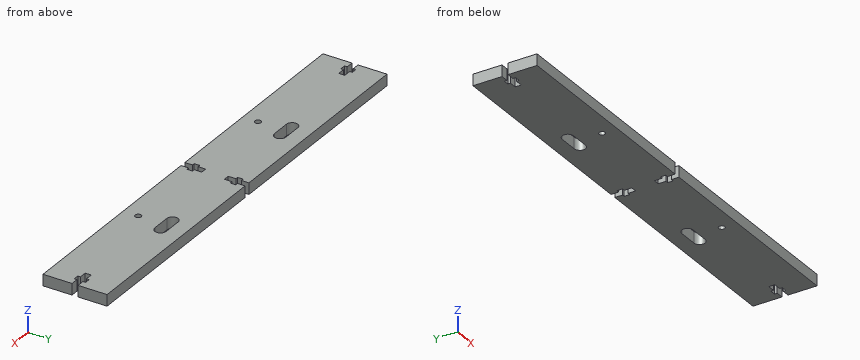
```python
from build123d import *

# Parameters (mm, degrees)
ESBO_O1_R                = 1.6
RESSALTO_EXTRUS_O1_DEPTH = 6


with BuildPart() as part:
    # Esboço1 → Ressalto-extrusão1 (new body)
    with BuildSketch(Plane.XY):
        Polygon((117, 17), (117, 1.6), (113, 1.6), (113, 3), (110, 3), (110, 1.6), (106, 1.6), (106, -1.6), (110, -1.6), (110, -3), (113, -3), (113, -1.6), (117, -1.6), (117, -17), (1.6, -17), (1.6, -13), (3, -13), (3, -10), (1.6, -10), (1.6, -6), (-1.6, -6), (-1.6, -10), (-3, -10), (-3, -13), (-1.6, -13), (-1.6, -17), (-117, -17), (-117, -1.6), (-113, -1.6), (-113, -3), (-110, -3), (-110, -1.6), (-106, -1.6), (-106, 1.6), (-110, 1.6), (-110, 3), (-113, 3), (-113, 1.6), (-117, 1.6), (-117, 17), (-1.6, 17), (-1.6, 13), (-3, 13), (-3, 10), (-1.6, 10), (-1.6, 6), (1.6, 6), (1.6, 10), (3, 10), (3, 13), (1.6, 13), (1.6, 17), align=None)
        with Locations((-50, -9)):
            Circle(ESBO_O1_R, mode=Mode.SUBTRACT)
        with Locations((50, -9)):
            Circle(ESBO_O1_R, mode=Mode.SUBTRACT)
        with BuildLine():
            Line((-55, 9), (-45, 9))
            ThreePointArc((-45, 9), (-42, 6), (-45, 3))
            Line((-45, 3), (-55, 3))
            ThreePointArc((-55, 3), (-58, 6), (-55, 9))
        make_face(mode=Mode.SUBTRACT)
        with BuildLine():
            Line((55, 9), (45, 9))
            ThreePointArc((45, 9), (42, 6), (45, 3))
            Line((45, 3), (55, 3))
            ThreePointArc((55, 3), (58, 6), (55, 9))
        make_face(mode=Mode.SUBTRACT)
    extrude(amount=RESSALTO_EXTRUS_O1_DEPTH)


solid = part.part
```
Check sheet for the modelled part. Datum: model origin and axes. Units: mm. Round coordinates to 2 decimals unless told otherwise and drop trailing zeros. Answer as a JSON object with one key per item and string values.
1. Gauge pin test, flat end, axial feed: P1, Ø1, axis at x = 0, z = 2, coming from the -Y side. Record the tip position at first contact, or that the pin passes through.
Reply:
{"P1": "stops at y = -6"}
2. Scan lines: line 1 (Y direction, x = 50, z = 1.7); line 2 (Y direction, x = 45, z = 0.9); line 3 (X direction, y = -12.5, z = 1.3). Record each from-to range of solid material in increasing order.
Reply:
{"line 1": "y = -17 to -10.6, -7.4 to 3, 9 to 17", "line 2": "y = -17 to 3, 9 to 17", "line 3": "x = -117 to -3, 3 to 117"}
3. Section check A-A (z = 3.8). State how many separate pieces and enclosed holes the cut face has, plus the area to 3 significant figures.
Reply:
{"separate pieces": "1", "enclosed holes": "4", "area": "7,590 mm²"}
